Check sheet for the modelled part. Datum: model origin and axes. Units: mm. Give positions to 0.01 mm unless a question says otherwise; leave off trailing zeros. Order: outer loops, then holes, each group sorted by start corner. A loop starts at its lowest first (then second) coordinate and runs counter-clockwise, first axis right, second up.
```python
from build123d import *

# Parameters (mm, degrees)
SKETCH_W                  = 152.4
SKETCH_H                  = 50.8
PAD_DEPTH                 = 12.7
SKETCH001_R               = 4.1021
POCKET_DEPTH              = 334.99087
SKETCH002_R               = 1.25
HOLE_DEPTH                = 334.99087
SKETCH002_MIRRORED001_2_R = 1.25
HOLE_MIRRORED001_2_DEPTH  = 334.99087


with BuildPart() as part:
    # Sketch → Pad (new body)
    with BuildSketch(Plane.XY):
        Rectangle(SKETCH_W, SKETCH_H)
    extrude(amount=-PAD_DEPTH)

    # Sketch001 (on Face5 of Pad) → Pocket (cut, through all)
    with BuildSketch(Plane.XY):
        with Locations((-63.5, 0)):
            Circle(SKETCH001_R)
    pocket = extrude(amount=-POCKET_DEPTH, mode=Mode.SUBTRACT)

    # Mirrored: Pocket across YZ
    add(pocket.mirror(Plane.YZ), mode=Mode.SUBTRACT)

    # Sketch002 (on Face4 of Mirrored) → Hole (cut, through all)
    with BuildSketch(Plane.XY):
        with Locations((12.95, 18.55)):
            Circle(SKETCH002_R)
    hole = extrude(amount=-HOLE_DEPTH, mode=Mode.SUBTRACT)

    # Sketch002 Mirrored001 2 → Hole Mirrored001 2 (cut, through all)
    with BuildSketch(Plane(origin=(0, 0, 0), x_dir=(-1, 0, 0), z_dir=(0, 0, -1))):
        with Locations((12.95, 18.55)):
            Circle(SKETCH002_MIRRORED001_2_R)
    hole_mirrored001_2 = extrude(amount=HOLE_MIRRORED001_2_DEPTH, mode=Mode.SUBTRACT)

    # Mirrored002: Hole, Hole Mirrored001 2 across XZ
    add(hole.mirror(Plane.XZ), mode=Mode.SUBTRACT)
    add(hole_mirrored001_2.mirror(Plane.XZ), mode=Mode.SUBTRACT)


solid = part.part
```
(1) Sectioned sample at B-B (y = 0). Enter the section's corners in (x, z).
(2) Sectioned sample at C-C (z = -9.5). Enter the section's corners in (x, y), plus the area to 3 significant figures.
(3) Thickness scan on L1, parallel to Y at x = -12.95, z = -8.5; L2, parallel to X at y = -18.55, z = -5; L3, parallel to Y at x = -63.5, z = -6.5. Record the ranges inside material, lowest first.
(4) Sectioned sample at A-A (x = 63.5). Enter the section's corners in (y, z).
(5) Go/stop test with flat-tipped pins: P1, Ø5, axis at x = -63.5, y = 0, coming from the +Z side; P2, Ø10, axis at x = 40.5, y = -5.5, coming from the +Z side. Record where each tip stops, or that it passes through.
(6) Sectioned sample at D-D (x = -62.5). Enter the section's corners in (y, z), plus the area to 3 significant figures.
Values follow:
1. outline: (-76.2, -12.7) - (-67.6, -12.7) - (-67.6, 0) - (-76.2, 0) - close; (-59.4, -12.7) - (59.4, -12.7) - (59.4, 0) - (-59.4, 0) - close; (67.6, -12.7) - (76.2, -12.7) - (76.2, 0) - (67.6, 0) - close
2. outline: (-76.2, -25.4) - (76.2, -25.4) - (76.2, 25.4) - (-76.2, 25.4) - close; hole circle Ø8.2 at (-63.5, 0); hole circle Ø2.5 at (-12.95, -18.55); hole circle Ø2.5 at (-12.95, 18.55); hole circle Ø2.5 at (12.95, -18.55); hole circle Ø2.5 at (12.95, 18.55); hole circle Ø8.2 at (63.5, 0)
2. area: 7,620 mm2
3. L1: y = -25.4 to -19.8, -17.3 to 17.3, 19.8 to 25.4
3. L2: x = -76.2 to -14.2, -11.7 to 11.7, 14.2 to 76.2
3. L3: y = -25.4 to -4.1, 4.1 to 25.4
4. outline: (-25.4, -12.7) - (-4.1, -12.7) - (-4.1, 0) - (-25.4, 0) - close; (4.1, -12.7) - (25.4, -12.7) - (25.4, 0) - (4.1, 0) - close
5. P1: passes through
5. P2: stops at z = 0
6. outline: (-25.4, -12.7) - (-3.98, -12.7) - (-3.98, 0) - (-25.4, 0) - close; (3.98, -12.7) - (25.4, -12.7) - (25.4, 0) - (3.98, 0) - close
6. area: 544 mm2
